Build history of the part. All positions in model axes, mm. A direction names the side the tool comes from. Give positions to 0.01 mm unless a question says otherwise; leave off trailing zeros. Order: outer loops, then holes, each group sorted by start corner. A loop starts at its lowest first (then second) coordinate and runs counter-clockwise, first axis right, second up. Notation, with made-up numbers: (56, 88) - (86, 88) arc R6 ccw to (86, 92) - close; hole circle Ø4 at (56, 80.5). An arc over 180 degrees is marked (long way). Use a Markdown table: item, result. Add a question column.
(1) Flat gauge pins, fed straight in: pin 1 (2 mm diameter, centred on y = 60, z = 19.5, fed in from +X); pin 2 (10 mm diameter, centred on x = -30, z = -24, fed in from +Y). Where does each tip first touch, or does it go through?
(2) Slice it at B-B (y = 92). Write the cut outline in (x, z).
(3) Which spindle directions (+Z, -Z, +X, -X, +Y, -Y) get a long thin tool onto all of the face, cutting with end or side? Do faces 1 (the face through (-1, 0, 1)), 2 (the face through (-50.2, 23.4, -50)). Say none if no direction does.
(4) Wall check: line 1 (X direction, y = 59, z = -37.5); line 2 (Y direction, x = 9, z = -10.5). Give the ranges that are in metal, low to high.
(5) Slice it at A-A (z = -38). Write the cut outline in (x, y).
(6) Slice it at C-C (x = -42). Write the cut outline in (y, z).
from build123d import *

# Parameters (mm, degrees)
F0_W     = 100
F0_H     = 100
F1_DEPTH = 6.35
F2_W     = 106.35
F2_H     = 100
F3_DEPTH = 6.35
F6_DEPTH = 25
F7_DEPTH = 25


with BuildPart() as f1:
    # F0 (on Front) → F1 (new body)
    with BuildSketch(Plane.XZ):
        Rectangle(F0_W, F0_H)
    extrude(amount=F1_DEPTH)

    # F2 (on face) → F3 (join)
    with BuildSketch(Plane(origin=(-50, 0, 0), x_dir=(0, -1, 0), z_dir=(-1, 0, 0))):
        with Locations((-46.825, 0)):
            Rectangle(F2_W, F2_H)
    extrude(amount=F3_DEPTH)

    # F5 (on face) → F6 (cut)
    with BuildSketch(Plane(origin=(-56.35, 0, 0), x_dir=(0, -1, 0), z_dir=(-1, 0, 0))):
        with BuildLine():
            Line((-100, 50), (-100, 10))
            ThreePointArc((-100, 10), (-71.715729, 21.715729), (-60, 50))
            Line((-60, 50), (-100, 50))
        make_face()
    extrude(amount=-F6_DEPTH, mode=Mode.SUBTRACT)

    # F4 (on face) → F7 (cut)
    with BuildSketch(Plane.XZ.offset(6.35)):
        with BuildLine():
            Line((50, 50), (10, 50))
            ThreePointArc((10, 50), (21.715729, 21.715729), (50, 10))
            Line((50, 10), (50, 50))
        make_face()
    extrude(amount=-F7_DEPTH, mode=Mode.SUBTRACT)


solid = f1.part
Solution:
| question | item | result |
|---|---|---|
| 1 | pin 1 | x = -50 |
| 1 | pin 2 | y = 0 |
| 2 | outline | (-56.35, -50) - (-50, -50) - (-50, 10.81) - (-56.35, 10.81) - close |
| 3 | face 1 | +Z, -Z, +X, +Y |
| 3 | face 2 | -Z, +X, -X, +Y, -Y |
| 4 | line 1 | -56.35 to -50 |
| 4 | line 2 | -6.35 to 0 |
| 5 | outline | (-56.35, -6.35) - (50, -6.35) - (50, 0) - (-50, 0) - (-50, 100) - (-56.35, 100) - close |
| 6 | outline | (-6.35, -50) - (0, -50) - (0, 50) - (-6.35, 50) - close |
